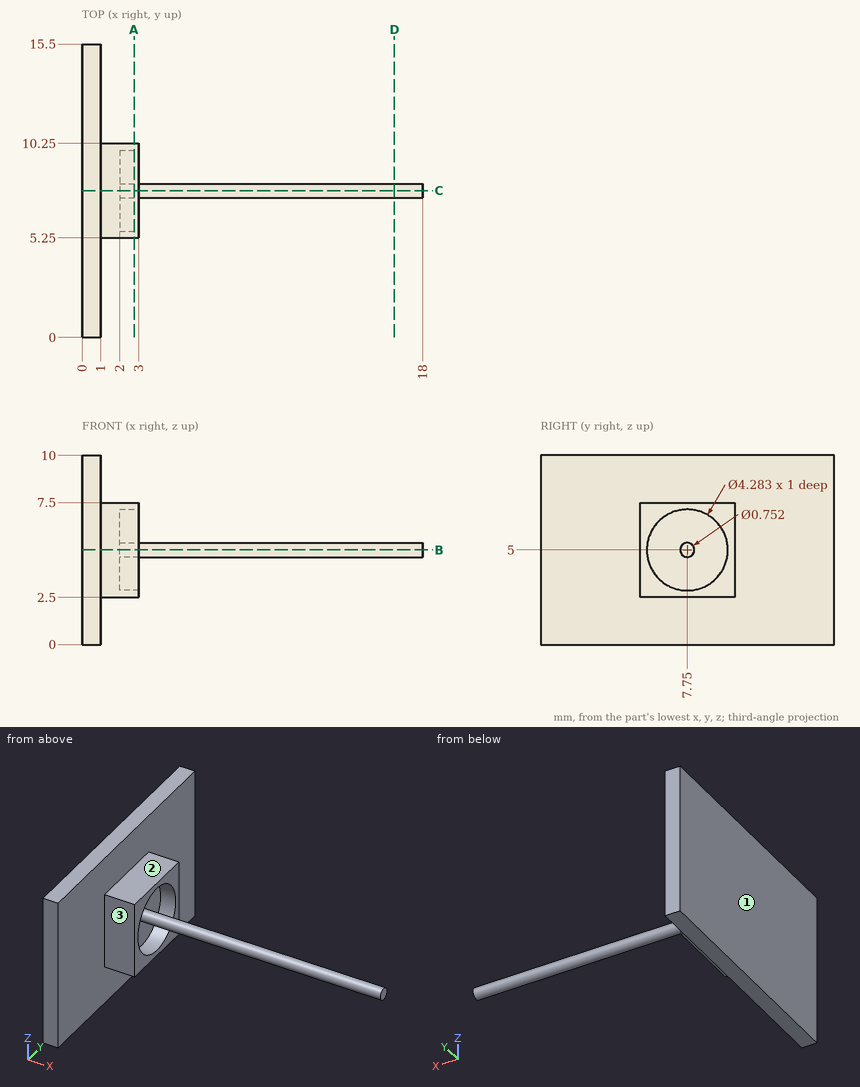
Answer from the drawing. Dimensions are ordinates in mm from the lowest x, y and z of the part. A direction names the side the tool comes from. Round coordinates to 2 decimals unless told otherwise and drop trailing zeros. Order: outer loops, then holes, each group sorted by start corner. A loop starts at its lowest first (then second) coordinate and runs counter-clockwise, first axis right, second up.
1) The part is cut by section B-B on z = 5. Write down the section's boundary in (x, y).
2) For the marked faces 1, 2 and 3, determine the directions among +Z, -Z, +X, -X, +Y, -Y from which every point of the face is accessible in a straight line to the end or side of a thin tool.
3) The part is cut by section A-A on x = 2.75. Write down the section's boundary in (y, z).
4) Straight lines are drawn through the part: L1, parallel to Y at x = 2.8, z = 5; L2, parallel to X at y = 3, z = 6.75. For each, find the intervals that lie inside material, in ascending order.
5) The part is cut by section D-D on x = 16.5. Write down the section's boundary in (y, z).
6) The part is cut by section C-C on y = 7.75. Write down the section's boundary in (x, z).
7) Flat-ended cylindrical pins translate along their axes: pin 1 (5 mm diameter, centred on x = 9.5, y = 12, fed in from -Z); pin 2 (1.6 mm diameter, centred on x = 2, z = 6, fed in from +Y); pin 3 (1 mm diameter, centred on x = 2.5, y = 7, fed in from -Z); pin 4 (2 mm diameter, centred on x = 6.5, y = 8.5, fed in from -Z). Find the tip coordinate at first contact, or state that the pin passes through.
Resolved:
1. outline: (0, 0) - (1, 0) - (1, 5.25) - (3, 5.25) - (3, 5.61) - (2, 5.61) - (2, 7.37) - (18, 7.37) - (18, 8.13) - (2, 8.13) - (2, 9.89) - (3, 9.89) - (3, 10.25) - (1, 10.25) - (1, 15.5) - (0, 15.5) - close
2. face 1: +Z, -Z, -X, +Y, -Y
2. face 2: +Z, +X, +Y, -Y
2. face 3: +Z, -Z, +X, -Y
3. outline: (5.25, 2.5) - (10.25, 2.5) - (10.25, 7.5) - (5.25, 7.5) - close; circle Ø0.75 at (7.75, 5); hole circle Ø4.28 at (7.75, 5)
4. L1: y = 5.25 to 5.61, 7.37 to 8.13, 9.89 to 10.25
4. L2: x = 0 to 1
5. outline: circle Ø0.75 at (7.75, 5)
6. outline: (0, 0) - (1, 0) - (1, 2.5) - (3, 2.5) - (3, 2.86) - (2, 2.86) - (2, 4.62) - (18, 4.62) - (18, 5.38) - (2, 5.38) - (2, 7.14) - (3, 7.14) - (3, 7.5) - (1, 7.5) - (1, 10) - (0, 10) - close
7. pin 1: passes through
7. pin 2: stops at y = 10.25
7. pin 3: stops at z = 2.5
7. pin 4: stops at z = 4.62
